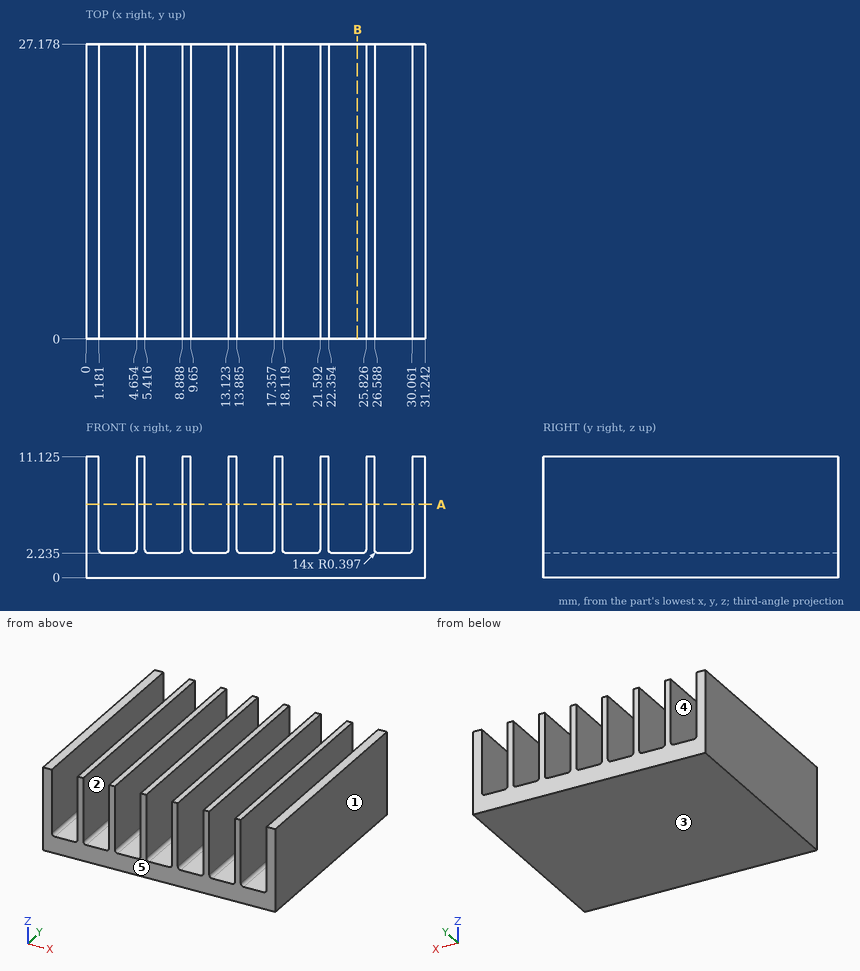
Here's the drawing with two shaded views (mm, measured from the low corner). I have some questions. A direction names the side the tool comes from. Round coordinates to 2 decimals unless told otherwise and drop trailing zeros. Order: outer loops, then holes, each group sorted by start corner. A loop starts at its lowest first (then second) coordinate and runs counter-clockwise, first axis right, second up. Notation, with made-up numbers: (-29, -32) -> (23, -32) arc R20 ccw to (23, -10) -> close; hole circle Ø5 at (-34.75, 48). An arc over 180 degrees is marked (long way). Use a Markdown table: item, result. Add a question column.
(1) Suppose I cut it at A-A, the plane z = 6.75. Count the separate pieces of the cut face and the enclosed holes in it.
(2) If we mould it in two halves opening along X, with no side actions, what happens to the marked faces 1, 2 and 3? For each: released by +X, released by -X, zero draft, split by the parting line, or undercut.
(3) For pin 1 Ø2 at (x, y) = (13, 9) entering from -Z; pin 2 Ø1.3 at (x, y) = (20.5, 19) entering from +Z (1 decimal), each with a flat end and sliding along its axis, tell me the tip position at first contact or that it passes through.
(4) Suppose I cut it at B-B, the plane x = 25. Please give me the cut outline in (y, z) (1 decimal).
(5) For the marked faces 4 and 5, which set-ups out of +Z, -Z, +X, -X, +Y, -Y let a thin tool reach every point of the face, with its end or its side?
(6) I need wall thicknesses on line 1 along Z through (x, y) = (25, 3) (1 decimal). Which ranges of the line are inside material? Lowest first, please.
Verdict:
| question | item | result |
|---|---|---|
| 1 | separate pieces | 8 |
| 1 | enclosed holes | 0 |
| 2 | face 1 | released by +X |
| 2 | face 2 | undercut |
| 2 | face 3 | zero draft |
| 3 | pin 1 | z = 0 |
| 3 | pin 2 | z = 2.2 |
| 4 | outline | (0, 0) -> (27.2, 0) -> (27.2, 2.2) -> (0, 2.2) -> close |
| 5 | face 4 | +Z, +Y, -Y |
| 5 | face 5 | +Z, -Z, +X, -X, -Y |
| 6 | line 1 | 0 to 2.2 |
